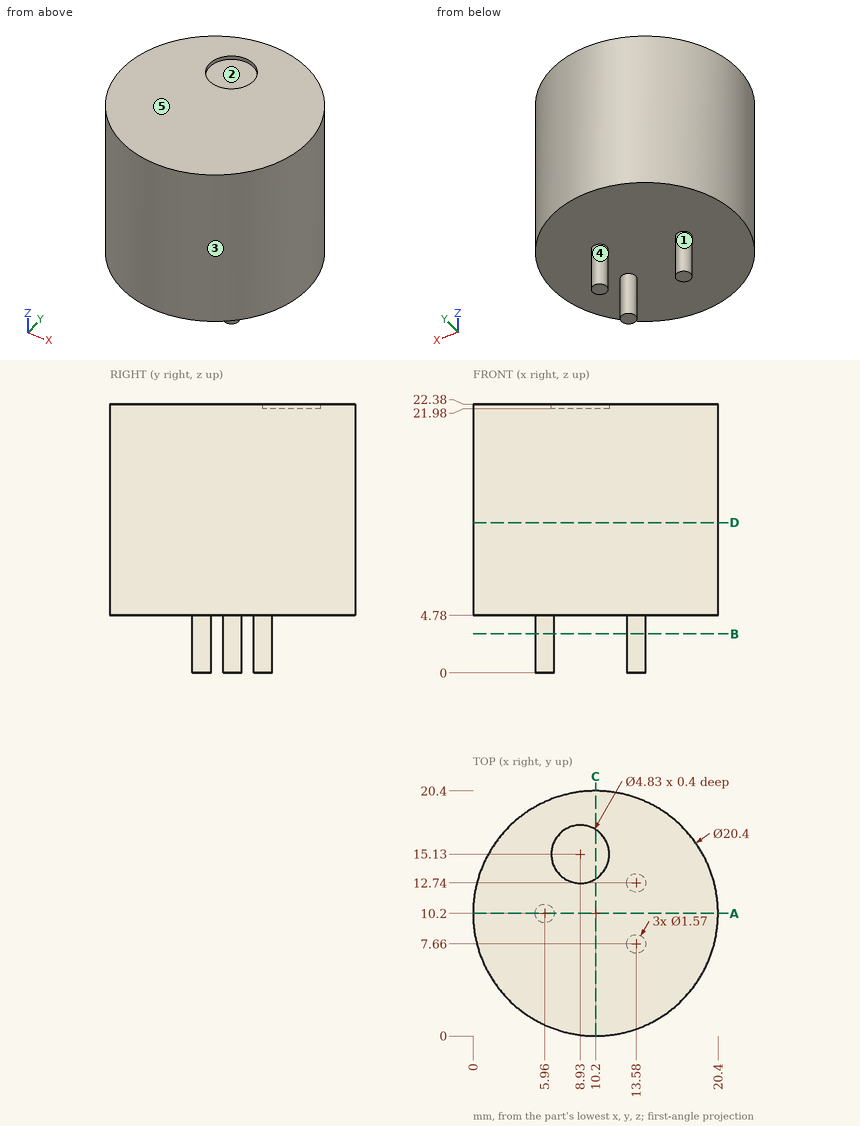
Source: three-view drawing plus pictorial views. Frame: mm from the lowest corner of the part. A direction names the side the tool comes from. Round coordinates to 2 decimals unless told otherwise and drop trailing zeros. Loops run counter-clockwise (first coordinate to the right, second up) from the corner with the lowest first, then second, coordinate; pieces in that order, holes last. Notation, with made-up numbers: (86.5, 39.5) -> (135.5, 39.5) arc R3 cw to (135.5, 43.5) -> close; hole circle Ø6 at (84.5, -25.75). An arc over 180 degrees is marked (long way). Use one line per item in the form item = value.
Item 1: Cut plane A-A on y = 10.2. Output: boundary loops of the cut face in (x, z) (3 decimals).
Evaluation:
outline = (0, 4.78) -> (5.175, 4.78) -> (5.175, 0) -> (6.745, 0) -> (6.745, 4.78) -> (20.4, 4.78) -> (20.4, 22.38) -> (0, 22.38) -> close
Item 2: Contact query for flat-ended pins moving along their axis: pin 1 Ø1 at (y, z) = (10, 4) entering from +X (3 decimals); pin 2 Ø1.5 at (x, z) = (17, 19.5) entering from +Y; pin 3 Ø2 at (y, z) = (4, 3) entering from -X; pin 4 Ø10 at (y, z) = (4.5, 4.5) entering from -X. Output: stop coordinate, or through.
Evaluation:
pin_1 = 6.745
pin_2 = 18.41
pin_3 = through
pin_4 = 0.02
Item 3: Cut plane D-D on z = 12.5. Output: boundary loops of the cut face in (x, y), then the cut area to 3 significant figures.
Evaluation:
outline = circle Ø20.4 at (10.2, 10.2)
area = 327 mm2
Item 4: Access query for the marked faces 1 and 2. Directions: +Z, -Z, +X, -X, +Y, -Y. A direction counts if a zero-diameter tool reaches every point of the face in a straight line with its end or side. Return the directions, or none.
Evaluation:
face_1 = -Z
face_2 = +Z
Item 5: Cut plane B-B on z = 3.25. Output: boundary loops of the cut face in (x, y) (3 decimals).
Evaluation:
outline = circle Ø1.57 at (5.96, 10.2); circle Ø1.57 at (13.58, 7.66); circle Ø1.57 at (13.58, 12.74)
Item 6: Cut plane C-C on x = 10.2. Output: boundary loops of the cut face in (y, z).
Evaluation:
outline = (0, 4.78) -> (20.4, 4.78) -> (20.4, 22.38) -> (17.18, 22.38) -> (17.18, 21.98) -> (13.08, 21.98) -> (13.08, 22.38) -> (0, 22.38) -> close
Item 7: Draft query along Y for the marked faces 3, 4 and 5. Return one class per face: released by +Y, released by -Y, zero draft, split by the parting line, or undercut.
Evaluation:
face_3 = split by the parting line
face_4 = undercut
face_5 = zero draft
Item 8: Material intervals for probe 1 along Z at (x, y) = (5, 5.5); probe 2 along Y at (x, z) = (8.93, 22.1) (3 decimals); probe 3 along X at (y, z) = (1.5, 18), sorted ascending.
Evaluation:
probe_1 = 4.78 to 22.38
probe_2 = 0.079 to 12.715, 17.545 to 20.321
probe_3 = 4.88 to 15.52
